The drawing under review shows one solid part. Ordinate dimensions are in mm from its lowest x, y, z. A direction names the side the tool comes from. Coordinates: 2 decimals unless noted, no trailing zeros. Order: outer loops, then holes, each group sorted by start corner. A loop starts at its lowest first (then second) coordinate and runs counter-clockwise, first axis right, second up. Notation, with made-up numbers: (-17.75, 56) -> (28.25, 56) arc R31 ccw to (28.25, 95) -> close; hole circle Ø6 at (69.25, 69). An arc over 180 degrees is marked (long way). Use a Markdown table: item, result. Add a question column.
Q1. Add section B-B (z = 14). State the section outline as (x, y) points.
Q2. Insertion check: pin 1 (5 mm diameter, centred on x = 12, z = 20.5, fed in from -Y); pin 2 (1.5 mm diameter, centred on x = 13, y = 11.5, fed in from -Z); pin 3 (4 mm diameter, centred on y = 23, z = 6, fed in from +X). Each pin has a flat end and moves straight along its axis. Give the tip position at first contact, or say it passes through.
Q3. Add section A-A (x = 14). State the section outline as (y, z) points.
Q4. Add section C-C (y = 18.5). State the section outline as (x, z) points, then the cut area to 3 significant figures.
Q5. Wall thickness on probe 1 along Y at (x, z) = (17.75, 8.5); probe 2 along Z at (x, y) = (14.5, 12); probe 3 along X at (y, z) = (12.5, 23.25): over which ranges is each line inside the solid? List them lowest first.
Q6. Machinability: for the marked faces 1 and 2, which of the approach directions +Z, -Z, +X, -X, +Y, -Y give a long, thin tool a straight path to every point of the face, cutting with its end or side? Answer none if there is none.
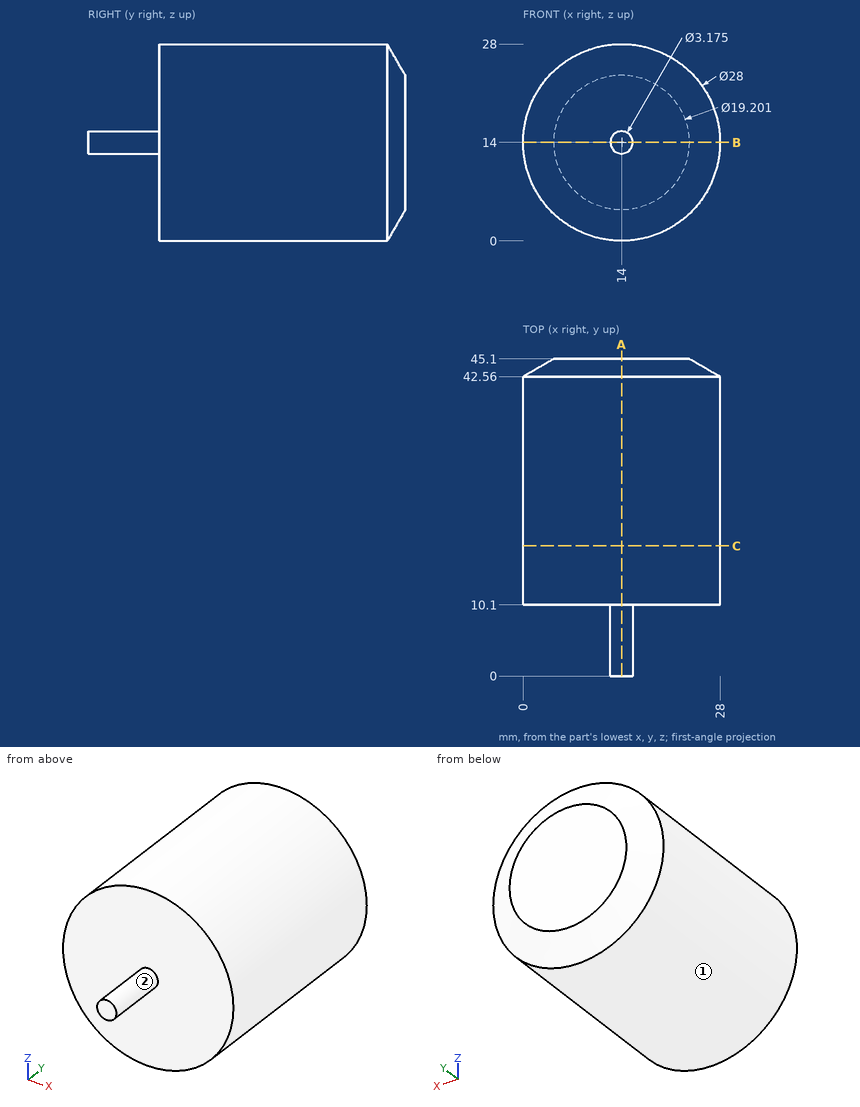
Established:
| question | item | result |
|---|---|---|
| 1 | outline | (0, 10.1) -> (12.41, 10.1) -> (12.41, 0) -> (15.59, 0) -> (15.59, 10.1) -> (28, 10.1) -> (28, 42.56) -> (23.6, 45.1) -> (4.4, 45.1) -> (0, 42.56) -> close |
| 2 | pin 1 | y = 10.1 |
| 2 | pin 2 | z = 0 |
| 2 | pin 3 | x = 26.65 |
| 3 | outline | (0, 12.41) -> (10.1, 12.41) -> (10.1, 0) -> (42.56, 0) -> (45.1, 4.4) -> (45.1, 23.6) -> (42.56, 28) -> (10.1, 28) -> (10.1, 15.59) -> (0, 15.59) -> close |
| 4 | outline | circle Ø28 at (14, 14) |
| 4 | area | 616 mm^2 |
| 5 | probe 1 | 10.1 to 45.1 |
| 5 | probe 2 | 0.01 to 27.99 |
| 5 | probe 3 | 3.49 to 24.51 |
| 6 | face 1 | +Y, -Y |
| 6 | face 2 | -Y |
